```python
from build123d import *

# Parameters (mm, degrees)
SKETCH1_W                   = 38.75
SKETCH1_H                   = 72.5
BOSS_EXTRUDE1_DEPTH         = 3.05
SKETCH4_W                   = 1.65
SKETCH4_H                   = 1
SKETCH4_H_2                 = 61.8
CUT_EXTRUDE1_DEPTH          = 76.106212293
SKETCH8_W                   = 38.75
SKETCH8_H                   = 8.3
CUT_EXTRUDE5_DEPTH          = 76.106212293
BOSS_EXTRUDE3_DEPTH         = 3.05
FILLET2_R                   = 0.5
TAP_DRILL_FOR_M3X0_5_TAP1_D = 2.5


with BuildPart() as part:
    # Sketch1 → Boss-Extrude1 (new body)
    with BuildSketch(Plane(origin=(0, 0, 0), x_dir=(1, 0, 0), z_dir=(0, 1, 0))):
        with Locations((0, 36.25)):
            Rectangle(SKETCH1_W, SKETCH1_H)
    extrude(amount=BOSS_EXTRUDE1_DEPTH)

    # Sketch4 → Cut-Extrude1 (cut, through all)
    with BuildSketch(Plane(origin=(0, 3.05, 0), x_dir=(1, 0, 0), z_dir=(0, 1, 0))):
        with Locations((-0.825, 70)):
            Rectangle(SKETCH4_W, SKETCH4_H)
        with Locations((-0.825, 37.4)):
            Rectangle(SKETCH4_W, SKETCH4_H_2)
        with Locations((0.825, 37.4)):
            Rectangle(SKETCH4_W, SKETCH4_H_2)
        with Locations((0.825, 70)):
            Rectangle(SKETCH4_W, SKETCH4_H)
    extrude(amount=-CUT_EXTRUDE1_DEPTH, mode=Mode.SUBTRACT)

    # Sketch8 → Cut-Extrude5 (cut, through all)
    with BuildSketch(Plane(origin=(0, 3.05, 0), x_dir=(1, 0, 0), z_dir=(0, 1, 0))):
        with Locations((0, 68.35)):
            Rectangle(SKETCH8_W, SKETCH8_H)
    extrude(amount=-CUT_EXTRUDE5_DEPTH, mode=Mode.SUBTRACT)

    # Sketch9 → Boss-Extrude3 (add)
    with BuildSketch(Plane(origin=(0, 3.05, 0), x_dir=(1, 0, 0), z_dir=(0, 1, 0))):
        Polygon((-14.7625, 66.2), (-13.375, 64.2), (-7.65, 64.2), (-6.2625, 66.2), align=None)
        Polygon((6.2625, 66.2), (7.65, 64.2), (13.375, 64.2), (14.7625, 66.2), align=None)
    extrude(amount=-BOSS_EXTRUDE3_DEPTH)

    # Fillet2
    fillet2_edges = [part.edges().sort_by_distance(p)[0] for p in [
        (14.7625, 1.525, -66.2),
        (13.375, 1.525, -64.2),
        (7.65, 1.525, -64.2),
        (6.2625, 1.525, -66.2),
        (-6.2625, 1.525, -66.2),
        (-7.65, 1.525, -64.2),
        (-13.375, 1.525, -64.2),
        (-14.7625, 1.525, -66.2),
    ]]
    fillet(fillet2_edges, radius=FILLET2_R)

    # Tap Drill for M3x0.5 Tap1 (through all)
    with Locations(Plane(origin=(0, 3.05, 0), x_dir=(1, 0, 0), z_dir=(0, 1, 0))):
        with Locations((-12, 3), (12, 3)):
            Hole(TAP_DRILL_FOR_M3X0_5_TAP1_D / 2)


solid = part.part
```
Check sheet for the modelled part. Datum: model origin and axes. Units: mm. A direction names the side the tool comes from. Coordinates: 2 decimals unless noted, no trailing zeros. Loops run counter-clockwise (first coordinate to the right, second up) from the corner with the lowest first, then second, coordinate; pieces in that order, holes last. Notation, with made-up numbers: M 68,70.25 L 90,70.25 A7 ccw 90,78.25 Z; hole C 65.25,26 d5. An arc over 180 degrees is marked long. Answer as a JSON object with one key per item and string values.
1. Sectioned sample at C-C on y = 2.4. Record the cut outline in (x, z) (3 decimals).
Outcome:
{"outline": "M -19.375,-64.2 L -14.33,-64.2 A0.5 cw -13.92,-64.985 L -14.218,-65.415 A0.5 ccw -13.807,-66.2 L -7.218,-66.2 A0.5 ccw -6.807,-65.415 L -7.105,-64.985 A0.5 cw -6.695,-64.2 L -1.65,-64.2 L -1.65,-6.5 L 1.65,-6.5 L 1.65,-64.2 L 6.695,-64.2 A0.5 cw 7.105,-64.985 L 6.807,-65.415 A0.5 ccw 7.218,-66.2 L 13.807,-66.2 A0.5 ccw 14.218,-65.415 L 13.92,-64.985 A0.5 cw 14.33,-64.2 L 19.375,-64.2 L 19.375,0 L -19.375,0 Z; hole C -12,-3 d2.5; hole C 12,-3 d2.5"}
2. Depth check by flat-ended pin: P1, Ø0.9, axis at x = 3.5, y = 1, coming from the -Z side. Enter the tip coordinate at first touch or a pass-through.
Outcome:
{"P1": "z = -64.2"}
3. Sectioned sample at B-B on z = -3. Record the cut outline in (x, y) (3 decimals), and give its area (3 significant figures).
Outcome:
{"outline": "M -19.375,0 L -13.25,0 L -13.25,3.05 L -19.375,3.05 Z; M -10.75,0 L 10.75,0 L 10.75,3.05 L -10.75,3.05 Z; M 13.25,0 L 19.375,0 L 19.375,3.05 L 13.25,3.05 Z", "area": "103 mm²"}
4. Access from +Z, -Z, +X, -X, +Y, -Y to the whole of each face (thin tool, end or side, straight path). Record for faces 1 (the flat face through (4, 2, -64.2)), 2 (the flat face through (-17, 2, -64.2)), 3 (the flat face through (19.375, 2, -32)), 4 (the flat face through (17, 2, -64.2)), 5 (the flat face through (11, 2, -66.2)).
Outcome:
{"face 1": "-Z, +Y, -Y", "face 2": "-Z, -X, +Y, -Y", "face 3": "+Z, -Z, +X, +Y, -Y", "face 4": "-Z, +X, +Y, -Y", "face 5": "-Z, +X, -X, +Y, -Y"}
5. Sectioned sample at A-A on x = -12. Record the cut outline in (y, z), and give its area (3 significant figures).
Outcome:
{"outline": "M 0,-66.2 L 3.05,-66.2 L 3.05,-4.25 L 0,-4.25 Z; M 0,-1.75 L 3.05,-1.75 L 3.05,0 L 0,0 Z", "area": "194 mm²"}
6. Release check for a two-part mould opening along Z. For faces 6 (the flat face through (-10, 2, -66.2)), 7 (the flat face through (0, 2, 0)), 8 (the cylindrical face through (12.921, 1.504, -3.845)) record: pulls with the +Z half, pulls with the -Z half, needs draft (parallel to the pull), parting line crosses it, or undercut.
Outcome:
{"face 6": "pulls with the -Z half", "face 7": "pulls with the +Z half", "face 8": "undercut"}
7. Sectioned sample at D-D on z = -58.5. Record the cut outline in (x, y) (3 decimals).
Outcome:
{"outline": "M -19.375,0 L -1.65,0 L -1.65,3.05 L -19.375,3.05 Z; M 1.65,0 L 19.375,0 L 19.375,3.05 L 1.65,3.05 Z"}
8. Scan lines: L1, parallel to X at y = 2, z = -10.5 (3 decimals); L2, parallel to Z at x = -12, y = 0.45; L3, parallel to X at y = 2, z = -4 (3 decimals). Record each from-to range of solid material in increasing order. Write a range as from..to.
Outcome:
{"L1": "-19.375..-1.65, 1.65..19.375", "L2": "-66.2..-4.25, -1.75..0", "L3": "-19.375..-12.75, -11.25..11.25, 12.75..19.375"}
